Design review of the part built by this model. Coordinates are the model's own, in mm. Coordinates: 2 decimals unless noted, no trailing zeros. Write each loop counter-clockwise with the first axis right and the second up, starting at its lowest first coordinate (ties: lowest second). Pieces come first, ordered by that corner, then holes.
Q1. Add section A-A, the plane x = -27.5. Give the boundary of the cut face in (y, z), plus the area to 3 significant figures.
Q2. Add section D-D, the plane y = 2.5. Give the number of separate pieces and of enclosed holes in the cut face, plus the area to 3 significant figures.
Q3. To check wall thickness, follow probe 1 along X at (y, z) = (4.75, 46.5) (3 decimals); probe 2 along X at (y, z) = (4.3, -80); probe 3 along X at (y, z) = (4.15, 72.5). State the ranges of each line that lie inside material, in increasing order.
Q4. Add section B-B, the plane z = 30. Give the boundary of the cut face in (x, y) (3 decimals).
Q5. Clearance check with flat-ended pins moving along their axes: pin 1 Ø1.4 at (y, z) = (2, 4) entering from +X; pin 2 Ø1.8 at (y, z) = (2.5, -57.5) entering from -X; pin 3 Ø1.8 at (x, y) = (23.5, 2.5) entering from -Z; pin 4 Ø5.5 at (x, z) = (-12.7, 69.95) entering from -Y. State where each tip first meets the part, or that it passes through.
Q6. Add section C-C, the plane x = 0. Give the boundary of the cut face in (y, z), plus the area to 3 significant figures.
from build123d import *

# Parameters (mm, degrees)
SKETCH1_R           = 3.175
SKETCH1_W           = 12.7
SKETCH1_H           = 5.842
BOSS_EXTRUDE1_DEPTH = 5.842
CUT_EXTRUDE1_DEPTH  = 116.299365115
FILLET1_R           = 1.5875
CUT_EXTRUDE2_DEPTH  = 116.299365115


with BuildPart() as part:
    # Sketch1 → Boss-Extrude1 (new body)
    with BuildSketch(Plane(origin=(0, 0, 0), x_dir=(1, 0, 0), z_dir=(0, 1, 0))):
        with BuildLine():
            Line((31.75, 26.724230903), (25.5, 26.724230903))
            Line((25.5, 26.724230903), (19.15, 26.724230903))
            Line((19.15, 26.724230903), (19.15, 32.566230903))
            Line((19.15, 32.566230903), (25.5, 32.566230903))
            Line((25.5, 32.566230903), (25.5, 74.730230903))
            Line((25.5, 74.730230903), (19.15, 74.730230903))
            Line((19.15, 74.730230903), (19.15, 80.572230903))
            Line((19.15, 80.572230903), (25.5, 80.572230903))
            Line((25.5, 80.572230903), (25.5, 88.9))
            Line((25.5, 88.9), (5.856060063, 104.213366787))
            ThreePointArc((5.856060063, 104.213366787), (0, 106.226230903), (-5.856060063, 104.213366787))
            Line((-5.856060063, 104.213366787), (-25.5, 88.9))
            Line((-25.5, 88.9), (-25.5, 80.572230903))
            Line((-25.5, 80.572230903), (-19.15, 80.572230903))
            Line((-19.15, 80.572230903), (-19.15, 74.730230903))
            Line((-19.15, 74.730230903), (-25.5, 74.730230903))
            Line((-25.5, 74.730230903), (-25.5, 32.566230903))
            Line((-25.5, 32.566230903), (-19.15, 32.566230903))
            Line((-19.15, 32.566230903), (-19.15, 26.724230903))
            Line((-19.15, 26.724230903), (-25.5, 26.724230903))
            Line((-25.5, 26.724230903), (-31.75, 26.724230903))
            Line((-31.75, 26.724230903), (-34.925, 26.724230903))
            Line((-34.925, 26.724230903), (-34.925, 32.566230903))
            Line((-34.925, 32.566230903), (-44.45, 32.566230903))
            Line((-44.45, 32.566230903), (-44.45, 26.724230903))
            Line((-44.45, 26.724230903), (-39.046137682, 0))
            Line((-39.046137682, 0), (-31.342, 0))
            Line((-31.342, 0), (-25.5, 0))
            Line((-25.5, 0), (-25.5, -18.542))
            Line((-25.5, -18.542), (-31.342, -18.542))
            Line((-31.342, -18.542), (-35.296790677, -18.542))
            Line((-35.296790677, -18.542), (-31.342, -38.1))
            Line((-31.342, -38.1), (-25.5, -38.1))
            Line((-25.5, -38.1), (-25.5, -56.642))
            Line((-25.5, -56.642), (-31.342, -56.642))
            Line((-31.342, -56.642), (-31.342, -69.342))
            Line((-31.342, -69.342), (-25.5, -69.342))
            Line((-25.5, -69.342), (-25.5, -85.217))
            Line((-25.5, -85.217), (25.5, -85.217))
            Line((25.5, -85.217), (25.5, -69.342))
            Line((25.5, -69.342), (31.342, -69.342))
            Line((31.342, -69.342), (31.342, -56.642))
            Line((31.342, -56.642), (25.5, -56.642))
            Line((25.5, -56.642), (25.5, -38.1))
            Line((25.5, -38.1), (31.342, -38.1))
            Line((31.342, -38.1), (35.296790677, -18.542))
            Line((35.296790677, -18.542), (31.342, -18.542))
            Line((31.342, -18.542), (25.5, -18.542))
            Line((25.5, -18.542), (25.5, 0))
            Line((25.5, 0), (31.342, 0))
            Line((31.342, 0), (39.046137682, 0))
            Line((39.046137682, 0), (44.45, 26.724230903))
            Line((44.45, 26.724230903), (44.45, 32.566230903))
            Line((44.45, 32.566230903), (34.925, 32.566230903))
            Line((34.925, 32.566230903), (34.925, 26.724230903))
            Line((34.925, 26.724230903), (31.75, 26.724230903))
        make_face()
        with Locations(Location((0, 96.701230903, 0), (0, 0, 270))):
            Circle(SKETCH1_R, mode=Mode.SUBTRACT)
        with Locations(Location((0, 57.053608903, 0), (0, 0, 270))):
            Circle(SKETCH1_R, mode=Mode.SUBTRACT)
        with Locations(Location((-12.7, -69.946391097, 0), (0, 0, 270))):
            Circle(SKETCH1_R, mode=Mode.SUBTRACT)
        with Locations(Location((12.7, -69.946391097, 0), (0, 0, 90))):
            Circle(SKETCH1_R, mode=Mode.SUBTRACT)
        with Locations((0, 77.651230903)):
            Rectangle(SKETCH1_W, SKETCH1_H, mode=Mode.SUBTRACT)
        with BuildLine():
            Line((9.525, -8.911080097), (9.525, -34.311080097))
            ThreePointArc((9.525, -34.311080097), (0, -43.836080097), (-9.525, -34.311080097))
            Line((-9.525, -34.311080097), (-9.525, -8.911080097))
            ThreePointArc((-9.525, -8.911080097), (0, 0.613919903), (9.525, -8.911080097))
        make_face(mode=Mode.SUBTRACT)
        with Locations((0, 29.645230903)):
            Rectangle(SKETCH1_W, SKETCH1_H, mode=Mode.SUBTRACT)
    extrude(amount=BOSS_EXTRUDE1_DEPTH)

    # Sketch2 → Cut-Extrude1 (cut, through all)
    with BuildSketch(Plane(origin=(0, 5.842, 0), x_dir=(1, 0, 0), z_dir=(0, 1, 0))):
        Polygon((-15.975, -42.6974), (-15.975, -41.402), (-19.15, -41.402), (-19.15, -42.6974), (-25.5, -42.6974), (-25.5, -46.2026), (-19.15, -46.2026), (-19.15, -47.498), (-15.975, -47.498), (-15.975, -46.2026), (-11.891999892, -46.2026), (-11.891999892, -42.6974), align=None)
        Polygon((-19.15, -8.1026), (-19.15, -9.398), (-15.975, -9.398), (-15.975, -8.1026), (-11.891999892, -8.1026), (-11.891999892, -4.5974), (-15.975, -4.5974), (-15.975, -3.302), (-19.15, -3.302), (-19.15, -4.5974), (-25.5, -4.5974), (-25.5, -8.1026), align=None)
        Polygon((15.975, -8.1026), (15.975, -9.398), (19.15, -9.398), (19.15, -8.1026), (25.5, -8.1026), (25.5, -4.5974), (19.15, -4.5974), (19.15, -3.302), (15.975, -3.302), (15.975, -4.5974), (11.891999892, -4.5974), (11.891999892, -8.1026), align=None)
        Polygon((19.15, -42.6974), (19.15, -41.402), (15.975, -41.402), (15.975, -42.6974), (11.891999892, -42.6974), (11.891999892, -46.2026), (15.975, -46.2026), (15.975, -47.498), (19.15, -47.498), (19.15, -46.2026), (25.5, -46.2026), (25.5, -42.6974), align=None)
    extrude(amount=-CUT_EXTRUDE1_DEPTH, mode=Mode.SUBTRACT)

    # Fillet1
    fillet1_edges = [part.edges().sort_by_distance(p)[0] for p in [
        (-25.5, 2.921, -88.9),
        (25.5, 2.921, -88.9),
    ]]
    fillet(fillet1_edges, radius=FILLET1_R)

    # Sketch3 → Cut-Extrude2 (cut, through all)
    with BuildSketch(Plane(origin=(0, 5.842, 0), x_dir=(1, 0, 0), z_dir=(0, 1, 0))):
        Polygon((-42.137472374, 23.29757819), (-39.620370832, 10.849518107), (-36.508355811, 11.478793492), (-39.025457353, 23.926853575), align=None)
        Polygon((39.025457353, 23.926853575), (36.508355811, 11.478793492), (39.620370832, 10.849518107), (42.137472374, 23.29757819), align=None)
    extrude(amount=-CUT_EXTRUDE2_DEPTH, mode=Mode.SUBTRACT)


solid = part.part
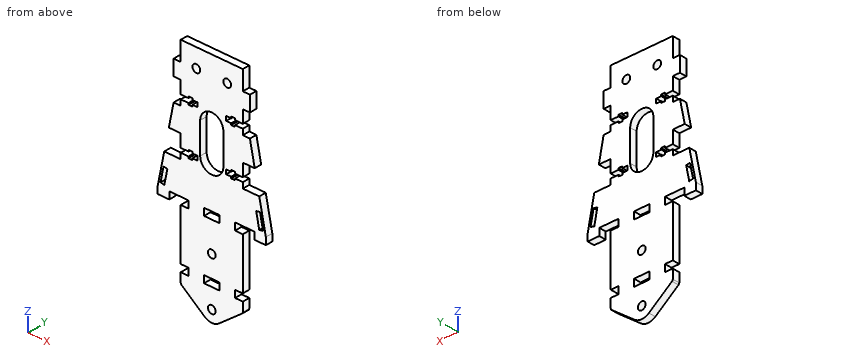
Here are the results:
1. outline: (0, -26.72) - (5.84, -26.72) - (5.84, 0) - (0, 0) - close; (0, 18.54) - (5.84, 18.54) - (5.84, 38.1) - (0, 38.1) - close; (0, 56.64) - (5.84, 56.64) - (5.84, 69.34) - (0, 69.34) - close
1. area: 345 mm2
2. separate pieces: 1
2. enclosed holes: 9
2. area: 9,310 mm2
3. probe 1: x = -25.5 to -19.15, -15.975 to 15.975, 19.15 to 25.5
3. probe 2: x = -19.15 to -6.35, 6.35 to 19.15
3. probe 3: x = -25.5 to -14.59, -10.81 to 10.81, 14.59 to 25.5
4. outline: (-32.98, 0) - (-9.525, 0) - (-9.525, 5.842) - (-32.98, 5.842) - close; (9.525, 0) - (32.98, 0) - (32.98, 5.842) - (9.525, 5.842) - close
5. pin 1: stops at x = 25.5
5. pin 2: stops at x = -25.5
5. pin 3: stops at z = -91.16
5. pin 4: passes through
6. outline: (0, -106.23) - (5.84, -106.23) - (5.84, -99.88) - (0, -99.88) - close; (0, -93.53) - (5.84, -93.53) - (5.84, -80.57) - (0, -80.57) - close; (0, -74.73) - (5.84, -74.73) - (5.84, -60.23) - (0, -60.23) - close; (0, -53.88) - (5.84, -53.88) - (5.84, -32.57) - (0, -32.57) - close; (0, -26.72) - (5.84, -26.72) - (5.84, -0.61) - (0, -0.61) - close; (0, 43.84) - (5.84, 43.84) - (5.84, 85.22) - (0, 85.22) - close
6. area: 716 mm2
